Verification items for this drawing (mm, ordinates from the low corner). Give positions to 0.01 mm unless a question says otherwise; leave off trailing zeros. Order: outer loops, then holes, each group sorted by start corner. A loop starts at its lowest first (then second) coordinate and runs counter-clockwise, first axis right, second up.
(1) Sectioned sample at A-A on x = 6. Record the cut outline in (y, z) (1 decimal).
(2) Scan lines: L1, parallel to Z at x = 16, y = 0.4 (1 decimal); L2, parallel to Z at x = 11.5, y = 0.7 (1 decimal); L3, parallel to X at y = 0.75, z = 1.25. Record each from-to range of solid material in increasing order.
(3) Sectioned sample at C-C on z = 14. Record the cut outline in (x, y).
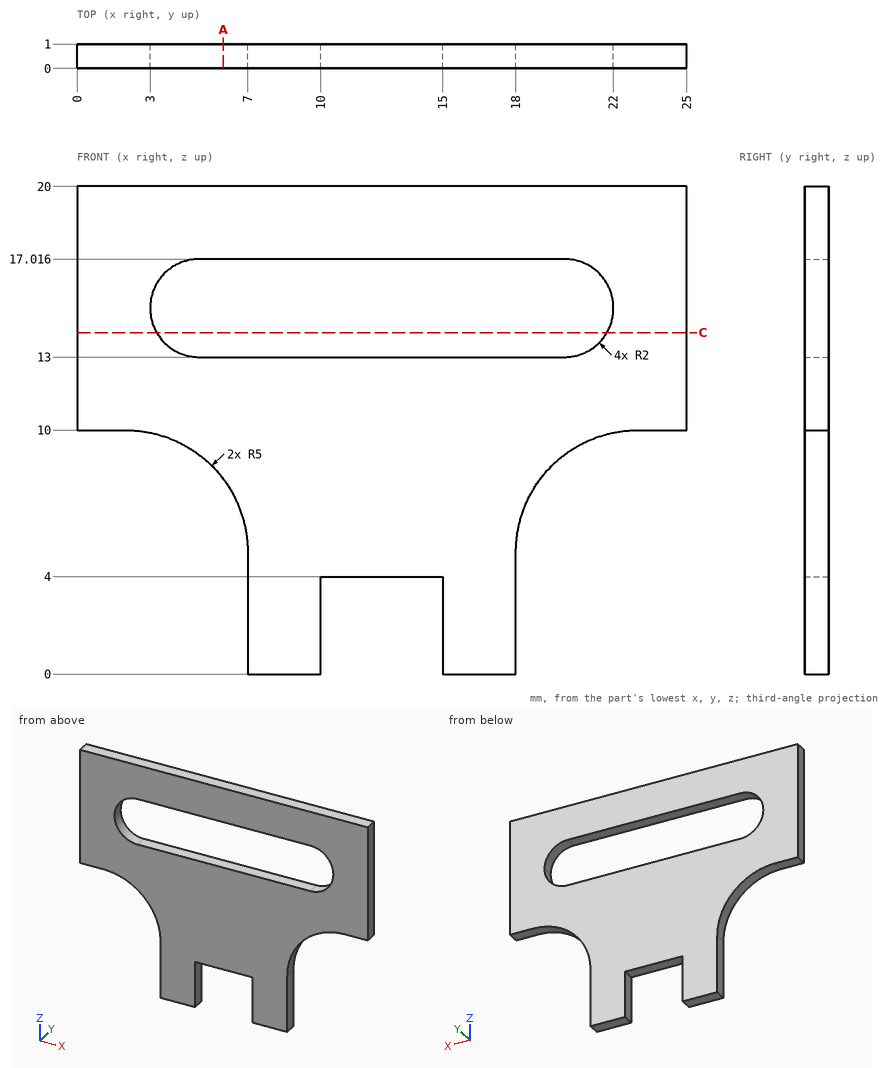
Ans:
1. outline: (0, 8) - (1, 8) - (1, 13) - (0, 13) - close; (0, 17) - (1, 17) - (1, 20) - (0, 20) - close
2. L1: z = 0 to 13, 17 to 20
2. L2: z = 4 to 13, 17 to 20
2. L3: x = 7 to 10, 15 to 18
3. outline: (0, 0) - (3.27, 0) - (3.27, 1) - (0, 1) - close; (21.73, 0) - (25, 0) - (25, 1) - (21.73, 1) - close
